Model file for the job. Use its own axes, mm. A direction names the side the tool comes from. Give positions to 0.01 mm unless a question says otherwise; leave off trailing zeros. Loops run counter-clockwise (first coordinate to the right, second up) from the corner with the lowest first, then second, coordinate; pieces in that order, holes last. Notation, with made-up numbers: (31, -13) - (70, -13) arc R15 ccw to (70, 5) - close; hole circle Ø8 at (-27, -2). An arc over 180 degrees is marked (long way). Use a Markdown table: item, result.
from build123d import *
from OCP.BRepFilletAPI import BRepFilletAPI_MakeChamfer

# Parameters (mm, degrees)
SKETCH1_W           = 1350
SKETCH1_H           = 250
BOSS_EXTRUDE1_DEPTH = 70
CHAMFER1_SIZE       = 10
CHAMFER1_SIZE2      = 20
SKETCH2_W           = 30
SKETCH2_H           = 250
BOSS_EXTRUDE2_DEPTH = 25
CHAMFER2_SIZE       = 20
FILLET1_R           = 10
SKETCH3_R           = 10
BOSS_EXTRUDE3_DEPTH = 25
CHAMFER3_SIZE       = 3


with BuildPart() as part:
    # Sketch1 → Boss-Extrude1 (new body)
    with BuildSketch(Plane(origin=(0, 0, 0), x_dir=(1, 0, 0), z_dir=(0, 1, 0))):
        Rectangle(SKETCH1_W, SKETCH1_H)
    extrude(amount=BOSS_EXTRUDE1_DEPTH)

    # Chamfer1: one chamfer whose edges measure the first distance from different faces: ONE call of the kernel's chamfer builder (chamfer() names one face for all edges)
    chamfer1_edges_1 = [part.edges().sort_by_distance(p)[0] for p in [
        (675, 70, 0),
    ]]
    chamfer1_side_1 = [part.faces().sort_by_distance(p)[0] for p in [
        (675, 35, 0),
    ]]
    chamfer1_edges_2 = [part.edges().sort_by_distance(p)[0] for p in [
        (0, 70, -125),
    ]]
    chamfer1_side_2 = [part.faces().sort_by_distance(p)[0] for p in [
        (0, 35, -125),
    ]]
    chamfer1_edges_3 = [part.edges().sort_by_distance(p)[0] for p in [
        (-675, 70, 0),
    ]]
    chamfer1_side_3 = [part.faces().sort_by_distance(p)[0] for p in [
        (-675, 35, 0),
    ]]
    chamfer1_edges_4 = [part.edges().sort_by_distance(p)[0] for p in [
        (0, 70, 125),
    ]]
    chamfer1_side_4 = [part.faces().sort_by_distance(p)[0] for p in [
        (0, 35, 125),
    ]]
    chamfer1 = BRepFilletAPI_MakeChamfer(part.part.solid().wrapped)
    for e in chamfer1_edges_1:
        chamfer1.Add(CHAMFER1_SIZE, CHAMFER1_SIZE2, e.wrapped, chamfer1_side_1[0].wrapped)  # the first distance lies on this face
    for e in chamfer1_edges_2:
        chamfer1.Add(CHAMFER1_SIZE, CHAMFER1_SIZE2, e.wrapped, chamfer1_side_2[0].wrapped)  # the first distance lies on this face
    for e in chamfer1_edges_3:
        chamfer1.Add(CHAMFER1_SIZE, CHAMFER1_SIZE2, e.wrapped, chamfer1_side_3[0].wrapped)  # the first distance lies on this face
    for e in chamfer1_edges_4:
        chamfer1.Add(CHAMFER1_SIZE, CHAMFER1_SIZE2, e.wrapped, chamfer1_side_4[0].wrapped)  # the first distance lies on this face
    add(Compound.cast(chamfer1.Shape()), mode=Mode.REPLACE)

    # Sketch2 → Boss-Extrude2 (add)
    with BuildSketch(Plane.XZ):
        with Locations((-90, 0)):
            Rectangle(SKETCH2_W, SKETCH2_H)
        with Locations((90, 0)):
            Rectangle(SKETCH2_W, SKETCH2_H)
    extrude(amount=BOSS_EXTRUDE2_DEPTH)

    # Chamfer2
    chamfer2_edges = [part.edges().sort_by_distance(p)[0] for p in [
        (-105, 0, 0),
        (105, 0, 0),
    ]]
    chamfer(chamfer2_edges, length=CHAMFER2_SIZE)

    # Fillet1
    fillet1_edges = [part.edges().sort_by_distance(p)[0] for p in [
        (-400, 0, -125),
        (675, 0, 0),
        (-125, 0, 0),
        (400, 0, -125),
        (400, 0, 125),
        (-400, 0, 125),
        (125, 0, 0),
        (-115, -10, -125),
        (-115, -10, 125),
        (115, -10, 125),
        (115, -10, -125),
        (-675, 0, 0),
    ]]
    fillet(fillet1_edges, radius=FILLET1_R)

    # Sketch3 → Boss-Extrude3 (add)
    with BuildSketch(Plane.XZ):
        with Locations(Location((0, 0, 0), (0, 0, 90))):
            Circle(SKETCH3_R)
    extrude(amount=BOSS_EXTRUDE3_DEPTH)

    # Chamfer3
    chamfer3_edges = [part.edges().sort_by_distance(p)[0] for p in [
        (0, -25, -10),
    ]]
    chamfer(chamfer3_edges, length=CHAMFER3_SIZE)


solid = part.part
(1) Slice it at B-B, the plane z = -32.5. Write the cut outline in (x, y).
Computed:
| item | result |
|---|---|
| outline | (-675, 10) arc R10 ccw to (-665, 0) - (-129.14, 0) arc R10 cw to (-122.07, -2.93) - (-105, -20) - (-105, -25) - (-75, -25) - (-75, 0) - (75, 0) - (75, -25) - (105, -25) - (105, -20) - (122.07, -2.93) arc R10 cw to (129.14, 0) - (665, 0) arc R10 ccw to (675, 10) - (675, 60) - (655, 70) - (-655, 70) - (-675, 60) - close |
(2) Slice it at A-A, the plane x = 344.5. Write the cut outline in (y, z).
Computed:
| item | result |
|---|---|
| outline | (0, -115) arc R10 ccw to (10, -125) - (60, -125) - (70, -105) - (70, 105) - (60, 125) - (10, 125) arc R10 ccw to (0, 115) - close |
(3) 3-axis set-ups, long thin cutter, end or side, ignore diameter. For faces 4 (the flat face through (-75, -12, -2)), 5 (the flat face through (-401, 0, -2)), 6 (the flat face through (393, 0, -2)): which of +Z, -Z, +X, -X, +Y, -Y reach the whole face in a straight line?
Computed:
| item | result |
|---|---|
| face 4 | +Z, -Z, -Y |
| face 5 | +Z, -Z, -X, -Y |
| face 6 | +Z, -Z, +X, -Y |
(4) Pin check, flat tips, straight feed: P1, Ø3, axis at x = 180, y = 0, coming from the -Z side; P2, Ø12.5, axis at y = -13, z = -4.5, coming from the +X side; P3, Ø15.5, axis at y = -18, z = 42, coming from the -X side. Stop position of each tip, or through.
Computed:
| item | result |
|---|---|
| P1 | z = -120.27 |
| P2 | x = 118.25 |
| P3 | x = -114.75 |
(5) Slice it at C-C, the plane x = -41. Write the cut outline in (y, z).
Computed:
| item | result |
|---|---|
| outline | (0, -125) - (60, -125) - (70, -105) - (70, 105) - (60, 125) - (0, 125) - close |
(6) Mould opens along X. For faces 1 (the flat face through (675, 35, 2)), 2 (the flat face through (-675, 35, 2)), 3 (the flat face through (75, -12, -2)) say: pulls with the +X half, pulls with the -X half, needs draft (parallel to the pull), parting line crosses it, or undercut.
Computed:
| item | result |
|---|---|
| face 1 | pulls with the +X half |
| face 2 | pulls with the -X half |
| face 3 | undercut |
(7) Drill centre lines: probe 1 along Y at (x, z) = (372, -79); probe 2 along X at (y, z) = (-2, -108.5); probe 3 along X at (y, z) = (-11.5, 31). Where is each one in solid material? Low to high. Write a range as [from, to].
Computed:
| item | result |
|---|---|
| probe 1 | [0, 70] |
| probe 2 | [-123.14, -75], [75, 123.14] |
| probe 3 | [-113.5, -75], [75, 113.5] |
